from build123d import *

# Parameters (mm, degrees)
CYLINDER014005857_R             = 2.15
CYLINDER014005857_DEPTH         = 16
CYLINDER014005858_R             = 3.6
CYLINDER014005858_DEPTH         = 4
FUSION001089095_PLACEMENT_ANGLE = 60
FUSION001089096_PLACEMENT_ANGLE = 120
FUSION001089097_PLACEMENT_ANGLE = 180
FUSION001089098_PLACEMENT_ANGLE = 240
FUSION001089099_PLACEMENT_ANGLE = 60
CYLINDER014005856_R             = 35
CYLINDER014005856_DEPTH         = 8


with BuildPart() as obj1:
    # Cylinder014005857 → Cylinder014005857 (new body)
    with BuildSketch(Plane(origin=(0, 24, -6), x_dir=(1, 0, 0), z_dir=(0, 0, 1))):
        Circle(CYLINDER014005857_R)
    extrude(amount=CYLINDER014005857_DEPTH)


with BuildPart() as obj2:
    # Cylinder014005858 → Cylinder014005858 (new body)
    with BuildSketch(Plane(origin=(0, 24, 6), x_dir=(1, 0, 0), z_dir=(0, 0, 1))):
        Circle(CYLINDER014005858_R)
    extrude(amount=CYLINDER014005858_DEPTH)

    # Fusion001089094: union obj1
    add(obj1.part)


with BuildPart() as obj3:
    # Fusion001089095 base: copy of obj2
    add(obj2.part)


with BuildPart() as obj3_1:
    # Fusion001089095 placement: moved
    add(obj3.part.rotate(Axis((0, 0, 0), (0, 0, 1)), FUSION001089095_PLACEMENT_ANGLE))


with BuildPart() as obj4:
    # Fusion001089096 base: copy of obj2
    add(obj2.part)


with BuildPart() as obj4_1:
    # Fusion001089096 placement: moved
    add(obj4.part.rotate(Axis((0, 0, 0), (0, 0, 1)), FUSION001089096_PLACEMENT_ANGLE))


with BuildPart() as obj5:
    # Fusion001089097 base: copy of obj2
    add(obj2.part)


with BuildPart() as obj5_1:
    # Fusion001089097 placement: moved
    add(obj5.part.rotate(Axis((0, 0, 0), (0, 0, 1)), FUSION001089097_PLACEMENT_ANGLE))


with BuildPart() as obj6:
    # Fusion001089098 base: copy of obj2
    add(obj2.part)


with BuildPart() as obj6_1:
    # Fusion001089098 placement: moved
    add(obj6.part.rotate(Axis((0, 0, 0), (0, 0, 1)), FUSION001089098_PLACEMENT_ANGLE))


with BuildPart() as obj7:
    # Fusion001089099 base: copy of obj2
    add(obj2.part)


with BuildPart() as obj7_1:
    # Fusion001089099 placement: moved
    add(obj7.part.rotate(Axis((0, 0, 0), (0, 0, -1)), FUSION001089099_PLACEMENT_ANGLE))


with BuildPart() as fusion001089100:
    # Fusion001089100 base: copy of obj2
    add(obj2.part)

    # Fusion001089100: union obj3, obj4, obj5, obj6, obj7
    add(obj3_1.part)
    add(obj4_1.part)
    add(obj5_1.part)
    add(obj6_1.part)
    add(obj7_1.part)


with BuildPart() as old:
    # Cylinder014005856 → Cylinder014005856 (new body)
    with BuildSketch(Plane.XY):
        Circle(CYLINDER014005856_R)
    extrude(amount=CYLINDER014005856_DEPTH)

    # Cut009003003008: cut Fusion001089100
    add(fusion001089100.part, mode=Mode.SUBTRACT)


solid = old.part
Can you work these out from the model? Positions are in its coordinate system, mm. A direction names the side the tool comes from. Round coordinates to 2 decimals unless told otherwise and drop trailing zeros. Write each loop counter-clockwise with the first axis right and the second up, starting at its lowest first coordinate (ties: lowest second). Pieces come first, ordered by that corner, then holes. Notation, with made-up numbers: (-5, 10.25) -> (8, 10.25) arc R18 ccw to (8, 26.25) -> close; hole circle Ø1 at (-2.75, 36.5). An arc over 180 degrees is marked (long way). One line per question, with ' | ' between items. Start each with the question number.
1) If we mould it in two halves opening along Y, with no side actions, what happens to faces 1 (the cylindrical face through (0.47, -21.9, 2.96)), 2 (the cylindrical face through (-28, -21, 4)), 3 (the flat face through (-2, -22, 6)), 4 (the flat face through (0, 0, 0))? For each: released by +Y, released by -Y, zero draft, split by the parting line, or undercut.
2) I'm going to push flat-ended pins straight in: P1, Ø4.5, axis at x = 20.78, y = -12, coming from the -Z side; P2, Ø3.5, axis at x = 20, y = -13.5, coming from the +Z side; P3, Ø1, axis at y = -17.5, z = 6, coming from the +X side; P4, Ø2, axis at x = -21, y = 11.5, coming from the +Z side. Where does each tip first touch, or does it pass through?
3) On a 3-axis mill with a long thin cutter (end or side, diameter ignored), from which of +Z, -Z, +X, -X, +Y, -Y can I reach the whole of each face in a straight line? I mean faces 5 (the cylindrical face through (-0.47, 27.57, 6.99)), 6 (the cylindrical face through (-18.637, 11.905, 2.958)). Say none if no direction works.
4) Suppose I cut it at C-C on z = 3.5. Write out the boundary of the cut face in (x, y), then the cut area to 3 significant figures.
5) Suppose I cut it at B-B on y = 12. Write out the boundary of the cut face in (x, z), then the cut area to 3 significant figures.
6) Suppose I cut it at D-D on y = -24. Write out the boundary of the cut face in (x, z).
7) Suppose I cut it at A-A on x = 0. Write out the boundary of the cut face in (y, z), then the cut area to 3 significant figures.
8) I need wall thicknesses on line 1 (Y direction, x = -1, z = 2.75); line 2 (X direction, y = 12.5, z = 5.25); line 3 (Y direction, x = 22.5, z = 7.25). Which ranges of each line are inside material? Lowest first, please. Write a range as [from, to].
Return value:
1) face 1: undercut | face 2: split by the parting line | face 3: undercut | face 4: zero draft
2) P1: stops at z = 0 | P2: stops at z = 6 | P3: stops at x = 30.59 | P4: passes through
3) face 5: +Z | face 6: +Z, -Z
4) outline: circle Ø70 at (0, 0); hole circle Ø4.3 at (-20.78, -12); hole circle Ø4.3 at (-20.78, 12); hole circle Ø4.3 at (0, -24); hole circle Ø4.3 at (0, 24); hole circle Ø4.3 at (20.78, -12); hole circle Ø4.3 at (20.78, 12) | area: 3,760 mm2
5) outline: (-32.88, 0) -> (-22.93, 0) -> (-22.93, 6) -> (-24.38, 6) -> (-24.38, 8) -> (-32.88, 8) -> close; (-18.63, 0) -> (18.63, 0) -> (18.63, 6) -> (17.18, 6) -> (17.18, 8) -> (-17.18, 8) -> (-17.18, 6) -> (-18.63, 6) -> close; (22.93, 0) -> (32.88, 0) -> (32.88, 8) -> (24.38, 8) -> (24.38, 6) -> (22.93, 6) -> close | area: 446 mm2
6) outline: (-25.48, 0) -> (-2.15, 0) -> (-2.15, 6) -> (-3.6, 6) -> (-3.6, 8) -> (-25.48, 8) -> close; (2.15, 0) -> (25.48, 0) -> (25.48, 8) -> (3.6, 8) -> (3.6, 6) -> (2.15, 6) -> close
7) outline: (-35, 0) -> (-26.15, 0) -> (-26.15, 6) -> (-27.6, 6) -> (-27.6, 8) -> (-35, 8) -> close; (-21.85, 0) -> (21.85, 0) -> (21.85, 6) -> (20.4, 6) -> (20.4, 8) -> (-20.4, 8) -> (-20.4, 6) -> (-21.85, 6) -> close; (26.15, 0) -> (35, 0) -> (35, 8) -> (27.6, 8) -> (27.6, 6) -> (26.15, 6) -> close | area: 480 mm2
8) line 1: y = [-34.99, -25.9], [-22.1, 22.1], [25.9, 34.99] | line 2: x = [-32.69, -22.88], [-18.69, 18.69], [22.88, 32.69] | line 3: y = [-26.81, -15.17], [-8.83, 8.83], [15.17, 26.81]
